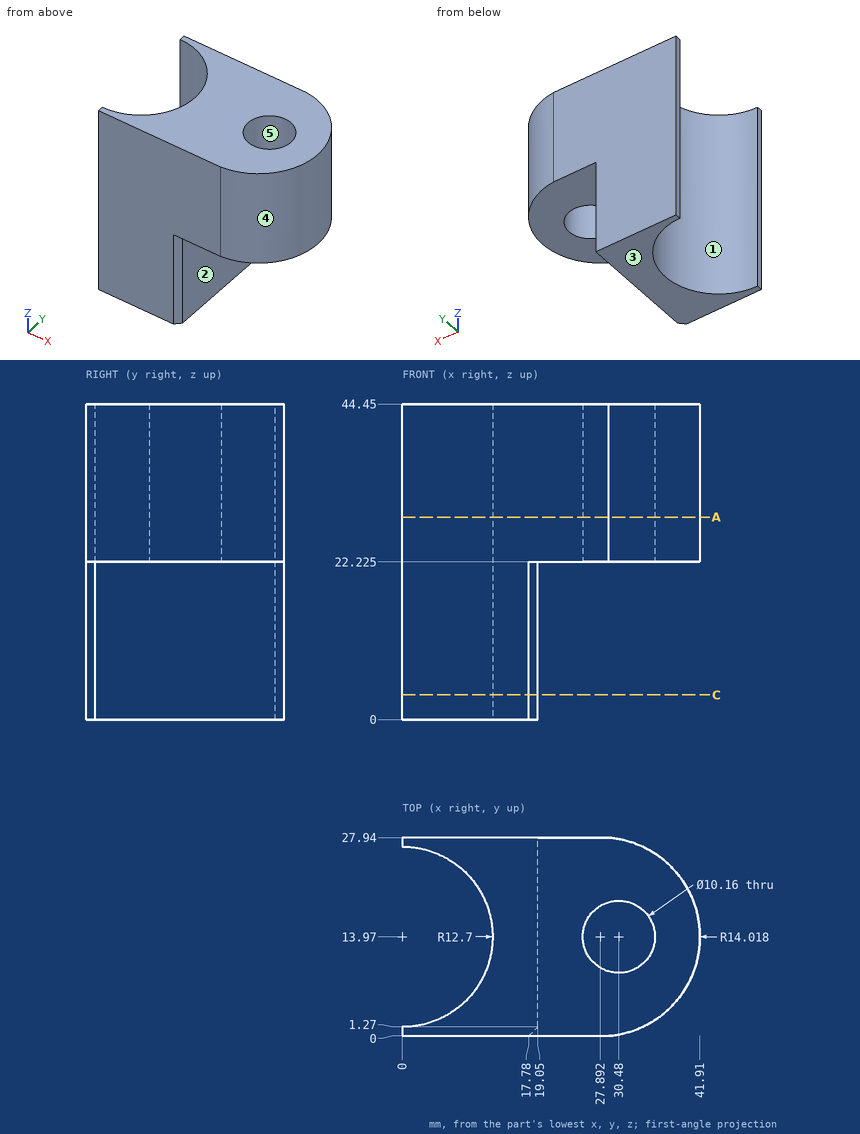
Geometry check sheet. Reference: drawing and pictorial views, mm from the part's lowest x, y, z. A direction names the side the tool comes from. Round coordinates to 2 decimals unless told otherwise and drop trailing zeros. Write each loop counter-clockwise with the first axis right and the second up, starting at its lowest first coordinate (ties: lowest second). Pieces come first, ordered by that corner, then holes.
Item 1: Access from +Z, -Z, +X, -X, +Y, -Y to the whole of each face (thin tool, end or side, straight path). Record for the marked faces 1 and 2.
Determined:
face 1: +Z, -Z, -X
face 2: -Z, +X, +Y, -Y
Item 2: Section check A-A (z = 28.5). Record the boundary of the cut face in (x, y) (1 decimal).
Determined:
outline: (0, 0) - (29, 0) arc R14 ccw to (29, 27.9) - (0, 27.9) - (0, 26.7) arc R12.7 cw to (0, 1.3) - close; hole circle Ø10.2 at (30.5, 14)
Item 3: Mould release check, pull along X, two halves, no side actions. Record for the marked faces 3, 4 and 5: +X half, -X half, draft (parallel to the pull), parting line (faces both ways), or undercut.
Determined:
face 3: draft
face 4: +X half
face 5: undercut
Item 4: Section check C-C (z = 3.5). Record the boundary of the cut face in (x, y).
Determined:
outline: (0, 0) - (17.78, 0) - (19.05, 1.27) - (19.05, 27.94) - (0, 27.94) - (0, 26.67) arc R12.7 cw to (0, 1.27) - close
Item 5: Go/stop test with flat-tipped pins: pin 1 Ø1 at (x, y) = (34.5, 23.5) entering from -Z (3 decimals); pin 2 Ø2 at (y, z) = (12.5, 12) entering from -X; pin 3 Ø10 at (y, z) = (6, 11) entering from +X; pin 4 Ø1.5 at (x, y) = (10, 13.5) entering from +Z. Record where each tip stops, or that it passes through.
Determined:
pin 1: stops at z = 22.225
pin 2: stops at x = 12.46
pin 3: stops at x = 19.05
pin 4: passes through
Item 6: Material ranges on line 1 along X through (y, z) = (11, 28.5); line 2 along Y through (x, z) = (2.5, 4); line 3 along Y through (x, z) = (30.48, 36.75), recorded low to high.
Determined:
line 1: x = 12.35 to 26.36, 34.6 to 41.59
line 2: y = 0 to 1.52, 26.42 to 27.94
line 3: y = 0.19 to 8.89, 19.05 to 27.75
